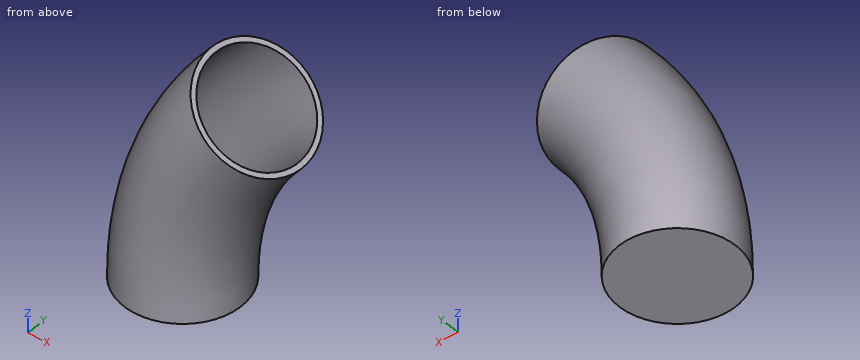
from build123d import *

# Parameters (mm, degrees)
F0_R          = 11.43
F3_DEPTH      = 11.4310001
F3_DEPTH_BACK = 11.4310001
F4_T          = -1


with BuildPart() as f1:
    # F0 (on Top) → F1 (revolve)
    with BuildSketch(Plane.XY):
        with Locations((-63.5, 0)):
            Circle(F0_R)
    revolve(axis=Axis((0, 30.6148057642, 0), (0, 1, 0)))

    # F2 (on Front) → F3 (cut, two sides)
    with BuildSketch(Plane.XZ) as f3_sk:
        with BuildLine():
            Line((-77.8301154209, 65.3072211442), (0, 0))
            Line((0, 0), (-101.6, 0))
            ThreePointArc((-101.6, 0), (95.4727702718, -34.7492465619), (-77.8301154209, 65.3072211442))
        make_face()
    extrude(amount=-F3_DEPTH, mode=Mode.SUBTRACT)
    extrude(f3_sk.sketch, amount=F3_DEPTH_BACK, mode=Mode.SUBTRACT)

    # F4
    f4_openings = [f1.faces().sort_by_distance(p)[0] for p in [
        (-48.643822, 0, 40.817013),
    ]]
    offset(amount=F4_T, openings=f4_openings)


solid = f1.part
For this review, take the finished solid that the model builds, in its own axes (mm). Round coordinates to 2 decimals unless told otherwise and drop trailing zeros. Order: outer loops, then holes, each group sorted by start corner. A loop starts at its lowest first (then second) coordinate and runs counter-clockwise, first axis right, second up. Notation, with made-up numbers: M 13.5,-22 L 67.5,-22 A22 ccw 67.5,3 Z; hole C -6,-2 d6. An arc over 180 degrees is marked long. Use a Markdown table: item, result. Add a question column.
Item 1: Insertion check: pin 1 (3 mm diameter, centred on x = -70, z = 7, fed in from -Y); pin 2 (6 mm diameter, centred on y = -9, z = 41.5, fed in from -X); pin 3 (3 mm diameter, centred on x = -59, z = 9, fed in from -Y). Each pin has a flat end and moves straight along its axis. Give the tip position at first contact, or say it passes through.
Item 2: Add section B-B, the plane y = 6. Give the boundary of the cut face in (x, z), then the cut area to 3 significant figures.
Item 3: Add section A-A, the plane y = 1.5. Give the boundary of the cut face in (x, z), then the cut area to 3 significant figures.
Item 4: To check wall thickness, follow line 1 along X through (y, z) = (2.25, 19.5); line 2 along X through (y, z) = (-5.5, 7); line 3 along Y through (x, z) = (-53.5, 33). State the ranges of each line that lie inside material, in increasing order.
Geometry results:
| question | item | result |
|---|---|---|
| 1 | pin 1 | stops at y = -10.1 |
| 1 | pin 2 | stops at x = -61.06 |
| 1 | pin 3 | stops at y = -11.19 |
| 2 | outline | M -73.23,0 L -53.77,0 A53.77 cw -41.19,34.56 L -42.11,35.33 A54.97 ccw -54.96,1 L -72.02,1 A72.03 cw -55.18,46.3 L -56.1,47.07 A73.23 ccw Z |
| 2 | area | 123 mm² |
| 3 | outline | M -74.83,0 L -52.17,0 A52.17 cw -39.96,33.53 L -40.74,34.18 A53.18 ccw -53.17,1 L -73.81,1 A73.82 cw -56.55,47.45 L -57.32,48.1 A74.83 ccw Z |
| 3 | area | 110 mm² |
| 4 | line 1 | x = -72.12 to -71.06, -49.62 to -48.52 |
| 4 | line 2 | x = -73.19 to -72.02, -54.19 to -53.02 |
| 4 | line 3 | y = -11.41 to -10.41, 10.41 to 11.41 |
